Check sheet for the modelled part. Datum: model origin and axes. Units: mm. A direction names the side the tool comes from. Round coordinates to 2 decimals unless told otherwise and drop trailing zeros. Order: outer loops, then holes, each group sorted by start corner. A loop starts at its lowest first (then second) coordinate and runs counter-clockwise, first axis right, second up. Notation, with made-up numbers: M 36,-9 L 78,-9 A13 ccw 78,3 Z; hole C -37,39 d3. An arc over 180 degrees is marked long. One line per item, written item: value. Start each with the question number.
(1) Depth check by flat-ended pin: pin 1 Ø7 at (x, y) = (-27.71, 16) entering from +Z; pin 2 Ø1.5 at (y, z) = (-10, 3) entering from +X; pin 3 Ø3 at (x, z) = (17.5, 7.5) entering from +Y. Enter the tip coordinate at first touch or a pass-through.
(2) Thickness scan on L1, parallel to Y at x = 0, z = 3; L2, parallel to X at y = 0, z = 2.3; L3, parallel to X at y = 16, z = 3. Record the ranges inside material, lowest first.
(3) Cross-section at B-B, the plane y = 0. Enter the section's corners in (x, z), and give its area (3 significant figures).
(4) Access from +Z, -Z, +X, -X, +Y, -Y to the whole of each face (thin tool, end or side, straight path). Record for faces 1 (the face through (10, -3, 5)), 2 (the face through (-0.52, 24.15, 10)), 3 (the face through (-25.717, -17.038, 4.93)).
(5) Cross-section at C-C, the plane z = 8. Enter the section's corners in (x, y), and give its area (3 significant figures).
(6) Release check for a two-part mould opening along Y. For faces 4 (the face through (-3.034, 9.634, 8.549)), 5 (the face through (1.055, -23.977, 10.74)), 6 (the face through (-1, 16, 0)) record: released by +Y, released by -Y, zero draft, split by the parting line, or undercut.
(7) Cross-section at A-A, the plane x = 0. Count the separate pieces of the cut face and the enclosed holes in it, and give its area (3 significant figures).
Autodesk Inventor part; units mm, degrees
ref_plane "YZ Plane" through (0, 0, 0) normal (1, 0, 0) x (0, 1, 0)
ref_plane "XZ Plane" through (0, 0, 0) normal (0, 1, 0) x (-1, 0, 0)
ref_plane "XY Plane" through (0, 0, 0) normal (0, 0, 1) x (1, 0, 0)
sketch "スケッチ1" plane through (0, 0, 0) normal (1, 0, 0) x (0, 1, 0)
  line L0 (12.1, 0) -> (12.1, 5)
  line L1 (12.1, 5) -> (10.1, 5)
  line L2 (10.1, 5) -> (10.1, 10)
  line L3 (37.5, 10) -> (37.5, 0)
  line L4 (37.5, 0) -> (12.1, 0)
  line L5 (0, -2.4) -> (0, 14.4)
  line L6 (10.1, 10) -> (10.1, 10)
  line L7 (10.1, 10) -> (10.1, 12)
  line L8 (10.1, 12) -> (24, 12)
  line L9 (24, 12) -> (24, 10)
  line L10 (24, 10) -> (37.5, 10)
  point P0 (0, 0)
  dimension "d0" = 12.1
  dimension "d1" = 37.5
  dimension "d2" = 2
  dimension "d3" = 5
  dimension "d5" = 10
  dimension "d31" = 24
  dimension "d32" = 2
  dimension "d34" = 0
revolve "回転1" add sketch "スケッチ1" angle 360 about axis through (0, 0, -10) along (0, 0, 1)
chamfer "面取り1" distance 0.5 angle 45 1 edges at (0, -12.1, 0)
sketch "スケッチ2" plane through (0, 0, 10) normal (0, 0, 1) x (1, 0, 0)
  circle A0 centre (0, 0) radius 32
  point P0 (0, 32)
  point P1 (-27.7128, 16)
  point P2 (-27.7128, -16)
  point P3 (0, -32)
  point P4 (27.7128, -16)
  point P5 (27.7128, 16)
  dimension "d10" = 64
  dimension "d13" = 360
hole "穴1" at (0, 32, 10) at (-27.7128, 16, 10) at (-27.7128, -16, 10) at (0, -32, 10) at (27.7128, -16, 10) at (27.7128, 16, 10) direction (0, 0, -1) diameter 4.5 end through all
chamfer "面取り2" distance 0.5 angle 45 2 edges at (0, -37.5, 0) (0, -37.5, 10)
chamfer "面取り3" distance 0.5 angle 45 1 edges at (0, -24, 12)
properties part number "unit-j2-base3" material "ABS プラスチック"
Values found:
1. pin 1: z = 10
1. pin 2: x = 36.34
1. pin 3: y = 33.92
2. L1: -37.5 to -34.25, -29.75 to -12.1, 12.1 to 29.75, 34.25 to 37.5
2. L2: -37.5 to -12.1, 12.1 to 37.5
2. L3: -33.92 to -29.96, -25.46 to 25.46, 29.96 to 33.92
3. outline: M -37.5,0.5 L -37,0 L -12.6,0 L -12.1,0.5 L -12.1,5 L -10.1,5 L -10.1,12 L -23.5,12 L -24,11.5 L -24,10 L -37,10 L -37.5,9.5 Z; M 10.1,5 L 12.1,5 L 12.1,0.5 L 12.6,0 L 37,0 L 37.5,0.5 L 37.5,9.5 L 37,10 L 24,10 L 24,11.5 L 23.5,12 L 10.1,12 Z
3. area: 583 mm^2
4. face 1: -Z
4. face 2: +Z
4. face 3: +Z, -Z
5. outline: C 0,0 d75; hole C -27.71,-16 d4.5; hole C -27.71,16 d4.5; hole C 0,0 d20.2; hole C 0,-32 d4.5; hole C 0,32 d4.5; hole C 27.71,-16 d4.5; hole C 27.71,16 d4.5
5. area: 4,000 mm^2
6. face 4: undercut
6. face 5: split by the parting line
6. face 6: zero draft
7. separate pieces: 4
7. enclosed holes: 0
7. area: 493 mm^2
